For this review, use the dimensioned drawing (mm, ordinates from the lowest corner) and the shaded views. Round coordinates to 2 decimals unless told otherwise and drop trailing zeros. Loops run counter-clockwise (first coordinate to the right, second up) from the corner with the lowest first, then second, coordinate; pieces in that order, holes last. Notation, with made-up numbers: M 85,-18.5 L 128,-18.5 A11 cw 128,-10.5 Z; hole C -33.5,63 d5. An arc over 180 degrees is marked long. One line per item, written item: value. Start each with the question number.
Item 1: We need section B-B (z = 21). Write out the cut boundary in (x, y), then the cut area to 3 significant figures.
Item 2: For line 1 along X through (y, z) = (2.1, 37.5) (1 decimal); line 2 along Z through (x, y) = (37, 1.5); line 3 along X through (y, z) = (2.1, 21.5), list the stretches that pass through material, from the lowest coordinate up.
Item 3: We need section A-A (x = 21). Write out the cut boundary in (y, z), then the cut area to 3 significant figures.
Item 4: We need section C-C (y = 1.3). Write out the cut boundary in (x, z).
Item 5: We need section D-D (x = 37). Write out the cut boundary in (y, z).
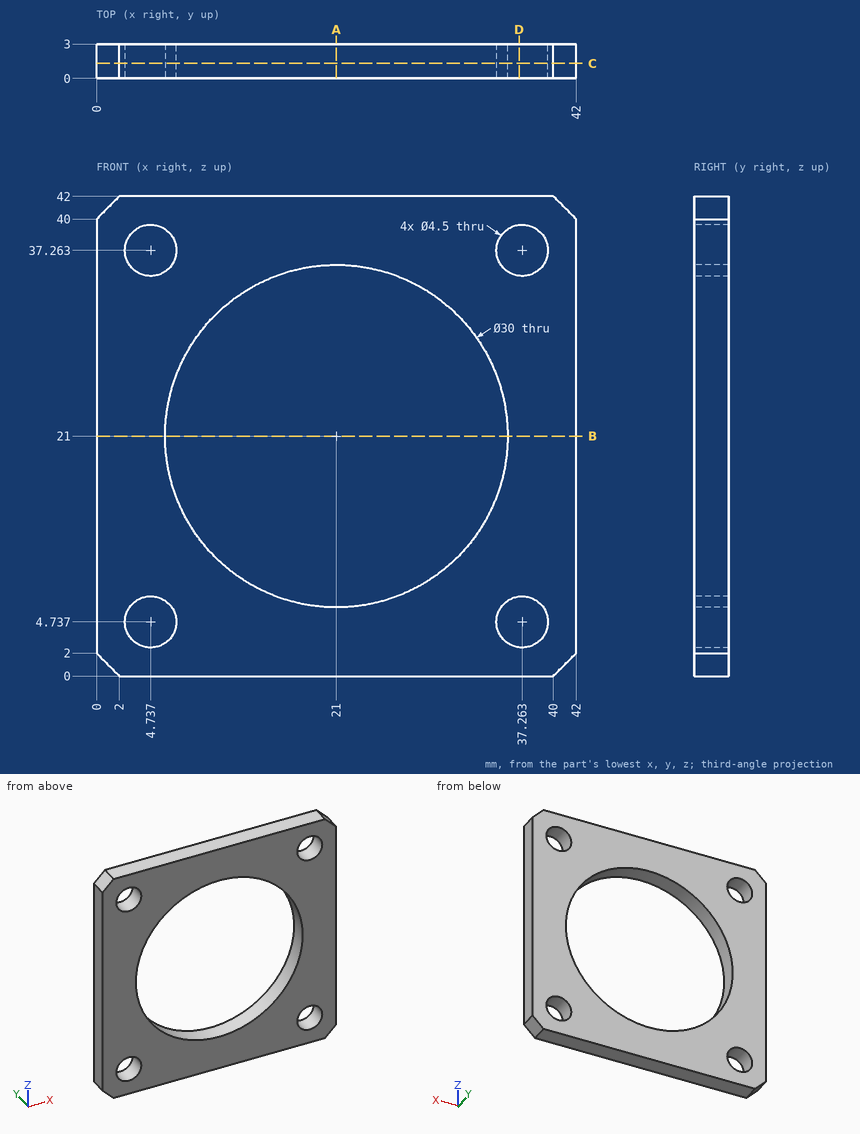
A:
1. outline: M 0,0 L 6,0 L 6,3 L 0,3 Z; M 36,0 L 42,0 L 42,3 L 36,3 Z
1. area: 36.0 mm2
2. line 1: 0 to 2.5, 7 to 35, 39.5 to 42
2. line 2: 0 to 2.5, 6.97 to 35.03, 39.5 to 42
2. line 3: 0 to 6.01, 35.99 to 42
3. outline: M 0,0 L 3,0 L 3,6 L 0,6 Z; M 0,36 L 3,36 L 3,42 L 0,42 Z
3. area: 36.0 mm2
4. outline: M 0,2 L 2,0 L 40,0 L 42,2 L 42,40 L 40,42 L 2,42 L 0,40 Z; hole C 4.74,4.74 d4.5; hole C 4.74,37.26 d4.5; hole C 21,21 d30; hole C 37.26,4.74 d4.5; hole C 37.26,37.26 d4.5
5. outline: M 0,0 L 3,0 L 3,2.5 L 0,2.5 Z; M 0,6.97 L 3,6.97 L 3,35.03 L 0,35.03 Z; M 0,39.5 L 3,39.5 L 3,42 L 0,42 Z
